```python
from build123d import *

# Parameters (mm, degrees)
F0_R      = 50.233177
F1_DEPTH  = 100.33
F1_FACE_R = 50.233177
F2_DEPTH  = 25.4
F3_R      = 19.910889
F4_DEPTH  = 258.826


with BuildPart() as f1:
    # F0 (on Top) → F1 (new body)
    with BuildSketch(Plane.XY):
        Circle(F0_R)
    extrude(amount=F1_DEPTH)

    # F1_face (on face) → F2 (cut)
    with BuildSketch(Plane.XY.offset(100.33)):
        Circle(F1_FACE_R)
    extrude(amount=-F2_DEPTH, mode=Mode.SUBTRACT)

    # F3 (on face) → F4 (cut)
    with BuildSketch(Plane.XY.offset(74.93)):
        with Locations((11.237776, -13.026105)):
            Circle(F3_R)
    extrude(amount=-F4_DEPTH, mode=Mode.SUBTRACT)


solid = f1.part
```
The listing builds one solid part. Answer for the finished solid, in the listing's coordinates (mm). Give positions to 0.01 mm unless a question says otherwise; leave off trailing zeros. Order: outer loops, then holes, each group sorted by start corner. A loop starts at its lowest first (then second) coordinate and runs counter-clockwise, first axis right, second up. Notation, with made-up numbers: M 29,-10.75 L 84,-10.75 A20 cw 84,19.25 Z; hole C 85.5,-39.5 d10. An arc over 180 degrees is marked long. Put each result on its own line as item: value. Start each with the question number.
Item 1: For a pull along Y with two mould halves and no side action, classify faces 1 (the face through (-1, 12, 0)), 2 (the face through (46.403, -19.24, 36.94)), 3 (the face through (30.23, -7.05, 37.99)) as +Y half, -Y half, draft (parallel to the pull), parting line (faces both ways), or undercut.
Item 2: The part is cut by section C-C, the plane z = 66.5. Determine the outline of the cut face in (x, y).
Item 3: The part is cut by section A-A, the plane y = 0. Determine the outline of the cut face in (x, z).
Item 4: The part is cut by section D-D, the plane y = -44. Determine the outline of the cut face in (x, z).
Item 5: Find the intervals of material crossed by line 1 along X through (y, z) = (-27.5, 15.5); line 2 along X through (y, z) = (-15, 23); line 3 along Y through (x, z) = (25, 21.5), in increasing order.
Item 6: The part is cut by section B-B, the plane x = 0.5. Determine the outline of the cut face in (y, z), and give its area (3 significant figures).
Item 7: Flat-ended cylindrical pins translate along their axes: P1, Ø10, axis at y = 30.5, z = 31, coming from the +X side; P2, Ø5, axis at x = 6.5, z = 28.5, coming from the -Y side; P3, Ø5, axis at x = -39.5, z = 57.5, coming from the +Y side. Find the tip coordinate at first contact, or state that the pin passes through.
Answer key:
1. face 1: draft
1. face 2: parting line
1. face 3: undercut
2. outline: C 0,0 d100.47; hole C 11.24,-13.03 d39.82
3. outline: M -50.23,0 L -3.82,0 L -3.82,74.93 L -50.23,74.93 Z; M 26.3,0 L 50.23,0 L 50.23,74.93 L 26.3,74.93 Z
4. outline: M -24.24,0 L 24.24,0 L 24.24,74.93 L -24.24,74.93 Z
5. line 1: x = -42.04 to -2.44, 24.91 to 42.04
5. line 2: x = -47.94 to -8.58, 31.05 to 47.94
5. line 3: y = -43.57 to -27.42, 1.36 to 43.57
6. outline: M -50.23,0 L -29.79,0 L -29.79,74.93 L -50.23,74.93 Z; M 3.74,0 L 50.23,0 L 50.23,74.93 L 3.74,74.93 Z
6. area: 5,010 mm²
7. P1: stops at x = 43.28
7. P2: stops at y = -50.07
7. P3: stops at y = 33.98
